```python
from build123d import *

# Parameters (mm, degrees)
BOSS_EXTRUDE1_DEPTH = 10
BOSS_EXTRUDE2_START = -2
BOSS_EXTRUDE2_DEPTH = 2
BOSS_EXTRUDE3_DEPTH = 2
SKETCH6_R           = 4.5
SKETCH6_R_2         = 2.9
BOSS_EXTRUDE4_DEPTH = 10
CUT_EXTRUDE1_START  = -8
SKETCH7_R           = 2.9
CUT_EXTRUDE1_DEPTH  = 8
SKETCH9_R           = 2.5
BOSS_EXTRUDE5_DEPTH = 10
BOSS_EXTRUDE6_START = -10
BOSS_EXTRUDE6_DEPTH = 10


with BuildPart() as part:
    # Sketch1 → Boss-Extrude1 (new body)
    with BuildSketch(Plane.XY):
        with BuildLine():
            Line((0, 0), (0, 15))
            Line((0, 15), (35, 15))
            Line((35, 15), (38.5, 18.724245534))
            Line((38.5, 18.724245534), (48.5, 18.724245534))
            Line((48.5, 18.724245534), (52, 15))
            Line((52, 15), (77.000664221, 15))
            Line((77.000664221, 15), (80.5, 18.723808414))
            Line((80.5, 18.723808414), (85.5, 18.723808414))
            Line((85.5, 18.723808414), (90.5, 18.723808414))
            Line((90.5, 18.723808414), (93.999335779, 15))
            Line((93.999335779, 15), (129, 15))
            Line((129, 15), (129, 0))
            Line((129, 0), (89, 0))
            ThreePointArc((89, 0), (85.5, 3.5), (82, 0))
            Line((82, 0), (47, 0))
            ThreePointArc((47, 0), (43.5, 3.5), (40, 0))
            Line((40, 0), (0, 0))
        make_face()
        with BuildLine():
            Line((2, 13), (35.865019983, 13))
            Line((35.865019983, 13), (39.365019983, 16.724245534))
            Line((39.365019983, 16.724245534), (47.634980017, 16.724245534))
            Line((47.634980017, 16.724245534), (51.134980017, 13))
            Line((51.134980017, 13), (77.865727104, 13))
            Line((77.865727104, 13), (81.365062883, 16.723808414))
            Line((81.365062883, 16.723808414), (85.5, 16.723808414))
            Line((85.5, 16.723808414), (89.634937117, 16.723808414))
            Line((89.634937117, 16.723808414), (93.134272896, 13))
            Line((93.134272896, 13), (127, 13))
            Line((127, 13), (127, 2))
            Line((127, 2), (90.623475383, 2))
            ThreePointArc((90.623475383, 2), (85.5, 5.5), (80.376524617, 2))
            Line((80.376524617, 2), (48.623475383, 2))
            ThreePointArc((48.623475383, 2), (43.5, 5.5), (38.376524617, 2))
            Line((38.376524617, 2), (2, 2))
            Line((2, 2), (2, 13))
        make_face(mode=Mode.SUBTRACT)
    extrude(amount=BOSS_EXTRUDE1_DEPTH)

    # Sketch2 → Boss-Extrude2 (add)
    with BuildSketch(Plane.XY.offset(10).offset(BOSS_EXTRUDE2_START)):
        with BuildLine():
            Line((129, 0), (129, 15))
            Line((129, 15), (93.999335779, 15))
            Line((93.999335779, 15), (90.5, 18.723808414))
            Line((90.5, 18.723808414), (80.5, 18.723808414))
            Line((80.5, 18.723808414), (77.000664221, 15))
            Line((77.000664221, 15), (52, 15))
            Line((52, 15), (48.5, 18.724245534))
            Line((48.5, 18.724245534), (38.5, 18.724245534))
            Line((38.5, 18.724245534), (35, 15))
            Line((35, 15), (0, 15))
            Line((0, 15), (0, 0))
            Line((0, 0), (40, 0))
            ThreePointArc((40, 0), (43.5, 3.5), (47, 0))
            Line((47, 0), (82, 0))
            ThreePointArc((82, 0), (85.5, 3.5), (89, 0))
            Line((89, 0), (129, 0))
        make_face()
    extrude(amount=BOSS_EXTRUDE2_DEPTH)

    # Sketch3 → Boss-Extrude3 (add)
    with BuildSketch(Plane(origin=(0, 0, 0), x_dir=(-1, 0, 0), z_dir=(0, 0, -1))):
        with BuildLine():
            Line((-52, 15), (-77.000664221, 15))
            Line((-77.000664221, 15), (-80.5, 18.723808414))
            Line((-80.5, 18.723808414), (-90.5, 18.723808414))
            Line((-90.5, 18.723808414), (-93.999335779, 15))
            Line((-93.999335779, 15), (-129, 15))
            Line((-129, 15), (-129, 0))
            Line((-129, 0), (-89, 0))
            ThreePointArc((-89, 0), (-85.5, 3.5), (-82, 0))
            Line((-82, 0), (-47, 0))
            ThreePointArc((-47, 0), (-43.5, 3.5), (-40, 0))
            Line((-40, 0), (0, 0))
            Line((0, 0), (0, 15))
            Line((0, 15), (-35, 15))
            Line((-35, 15), (-38.5, 18.724245534))
            Line((-38.5, 18.724245534), (-48.5, 18.724245534))
            Line((-48.5, 18.724245534), (-52, 15))
        make_face()
    extrude(amount=-BOSS_EXTRUDE3_DEPTH)

    # Sketch6 → Boss-Extrude4 (add)
    with BuildSketch(Plane.XY.offset(10)):
        with Locations(Location((64.500332111, 7.717300047, 0), (0, 0, 180))):
            Circle(SKETCH6_R)
        with Locations((64.500332111, 7.717300047)):
            Circle(SKETCH6_R_2, mode=Mode.SUBTRACT)
    extrude(amount=BOSS_EXTRUDE4_DEPTH)

    # Sketch7 → Cut-Extrude1 (cut)
    with BuildSketch(Plane.XY.offset(10).offset(CUT_EXTRUDE1_START)):
        with Locations((64.500332111, 7.717300047)):
            Circle(SKETCH7_R)
    extrude(amount=CUT_EXTRUDE1_DEPTH, mode=Mode.SUBTRACT)

    # Sketch9 → Boss-Extrude5 (add)
    with BuildSketch(Plane.XY.offset(10)):
        with Locations((119, 7.5)):
            Circle(SKETCH9_R)
        with Locations((103, 7.5)):
            Circle(SKETCH9_R)
        with Locations((76.500332111, 7.5)):
            Circle(SKETCH9_R)
        with Locations((10.000664221, 7.5)):
            Circle(SKETCH9_R)
        with Locations((26.000664221, 7.5)):
            Circle(SKETCH9_R)
        with Locations((52.500332111, 7.5)):
            Circle(SKETCH9_R)
    extrude(amount=-BOSS_EXTRUDE5_DEPTH)

    # Sketch10 → Boss-Extrude6 (add)
    with BuildSketch(Plane.XY.offset(20).offset(BOSS_EXTRUDE6_START)):
        with BuildLine():
            Line((60.000332111, 7.717300047), (60.000332111, 0))
            Line((60.000332111, 0), (69.000332111, 0))
            Line((69.000332111, 0), (69.000332111, 7.717300047))
            ThreePointArc((69.000332111, 7.717300047), (64.500332111, 3.217300047), (60.000332111, 7.717300047))
        make_face()
    extrude(amount=BOSS_EXTRUDE6_DEPTH)


solid = part.part
```
Work out the finished part from the listing and answer in its coordinate system (mm). A direction names the side the tool comes from. Round coordinates to 2 decimals unless told otherwise and drop trailing zeros. Write each loop counter-clockwise with the first axis right and the second up, starting at its lowest first coordinate (ties: lowest second). Pieces come first, ordered by that corner, then holes. Notation, with made-up numbers: (38.5, 55) - (87.5, 55) arc R23 ccw to (87.5, 80) - close; hole circle Ø3 at (69, 80). An arc over 180 degrees is marked (long way). Return JSON: item names as keys, results as strings. Group by question number.
Q1. The part is cut by section C-C on x = 103. Write down the section's boundary in (y, z).
Q2. The mould has two halves that part along Y. Classify faces 4 (the flat face through (17, 15, 5)), 5 (the flat face through (65, 7, 0)), 6 (the flat face through (109, 0, 5)), 7 (the flat face through (109, 2, 5)): released by +Y, released by -Y, zero draft, split by the parting line, or undercut.
Q3. For faces 1 (the flat face through (64, 15, 5)), 2 (the cylindrical face through (105.385, 8.251, 5.042)), 3 (the flat face through (43, 18.724, 5)), determine the directions among +Z, -Z, +X, -X, +Y, -Y from which every point of the face is accessible in a straight line to the end or side of a thin tool.
Q4. The part is cut by section B-B on z = 13.5. Write down the section's boundary in (x, y), then the cut area to 3 significant figures.
Q5. The part is cut by section D-D on x = 43.5. Write down the section's boundary in (y, z).
Q6. Find the intervals of material crossed by L1, parallel to Z at x = 71, y = 9; L2, parallel to X at y = 14, z = 3.5; L3, parallel to X at y = 11.75, z = 6.25, in increasing order.
Q7. The part is cut by section A-A on x = 30. Write down the section's boundary in (y, z).
Q8. Each of these flat-tipped pins is pushed along its axis until it touches: pin 1 Ø8.5 at (y, z) = (2, 16) entering from -X; pin 2 Ø8 at (y, z) = (11.5, 16.5) entering from +X; pin 3 Ø11 at (x, z) = (9.5, 4.5) entering from +Y. Where does it stop, or does it pass through?
Solved:
{
 "1": {"outline": "(0, 0) - (15, 0) - (15, 10) - (0, 10) - close; hole (2, 2) - (5, 2) - (5, 8) - (2, 8) - close; hole (10, 2) - (13, 2) - (13, 8) - (10, 8) - close"},
 "2": {"face 4": "released by +Y", "face 5": "zero draft", "face 6": "released by -Y", "face 7": "undercut"},
 "3": {"face 1": "+Z, -Z, +Y", "face 2": "none", "face 3": "+Z, -Z, +X, -X, +Y"},
 "4": {"outline": "(60, 0) - (69, 0) - (69, 7.72) arc R4.5 ccw to (60, 7.72) - close; hole circle Ø5.8 at (64.5, 7.72)", "area": "74.8 mm²"},
 "5": {"outline": "(3.5, 0) - (18.72, 0) - (18.72, 10) - (3.5, 10) - close; hole (5.5, 2) - (16.72, 2) - (16.72, 8) - (5.5, 8) - close"},
 "6": {"L1": "0 to 2, 8 to 10", "L2": "0 to 36.8, 50.2 to 78.81, 92.19 to 129", "L3": "0 to 2, 127 to 129"},
 "7": {"outline": "(0, 0) - (15, 0) - (15, 10) - (0, 10) - close; hole (2, 2) - (13, 2) - (13, 8) - (2, 8) - close"},
 "8": {"pin 1": "x = 60", "pin 2": "x = 69", "pin 3": "y = 15"}
}
